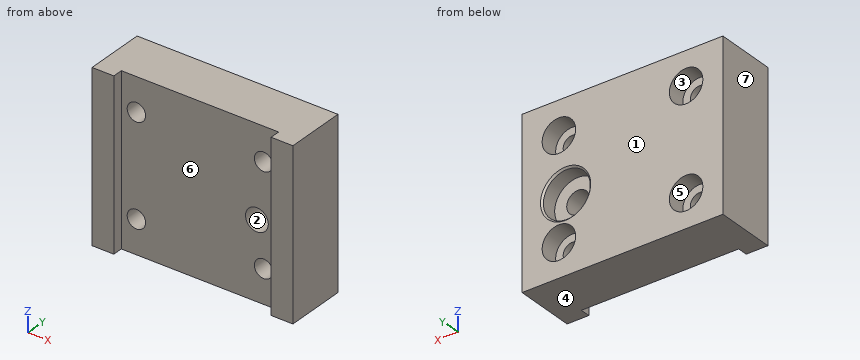
from build123d import *

# Parameters (mm, degrees)
SKETCH1_W                                           = 60
SKETCH1_H                                           = 50
BOSS_EXTRUDE1_DEPTH                                 = 9
SKETCH2_W                                           = 47
SKETCH2_H                                           = 6
CUT_EXTRUDE1_DEPTH                                  = 60
CBORE_FOR_M5_HEX_SOCKET_HEAD_CAP_SCREW1_D           = 5.5
CBORE_FOR_M5_HEX_SOCKET_HEAD_CAP_SCREW1_CBORE_D     = 10
CBORE_FOR_M5_HEX_SOCKET_HEAD_CAP_SCREW1_CBORE_DEPTH = 5.4
M8_TAPPED_HOLE1_D                                   = 6.8
SKETCH9_R                                           = 7
CUT_EXTRUDE2_DEPTH                                  = 5
CHAMFER1_SIZE                                       = 0.5


with BuildPart() as part:
    # Sketch1 → Boss-Extrude1 (new, symmetric)
    with BuildSketch(Plane(origin=(0, 0, 0), x_dir=(1, 0, 0), z_dir=(0, 1, 0))):
        Rectangle(SKETCH1_W, SKETCH1_H)
    extrude(amount=BOSS_EXTRUDE1_DEPTH, both=True)

    # Sketch2 → Cut-Extrude1 (cut, through all)
    with BuildSketch(Plane.XY.offset(25)):
        with Locations((0, -9)):
            Rectangle(SKETCH2_W, SKETCH2_H)
    extrude(amount=-CUT_EXTRUDE1_DEPTH, mode=Mode.SUBTRACT)

    # CBORE for M5 Hex Socket Head Cap Screw1 (through all)
    with Locations(Plane(origin=(0, 9, 0), x_dir=(1, 0, 0), z_dir=(0, 1, 0))):
        with Locations((-19, 15), (19, 15), (19, -15), (-19, -15)):
            CounterBoreHole(CBORE_FOR_M5_HEX_SOCKET_HEAD_CAP_SCREW1_D / 2, CBORE_FOR_M5_HEX_SOCKET_HEAD_CAP_SCREW1_CBORE_D / 2, CBORE_FOR_M5_HEX_SOCKET_HEAD_CAP_SCREW1_CBORE_DEPTH)

    # M8 Tapped Hole1 (through all)
    with Locations(Plane(origin=(0, 9, 0), x_dir=(1, 0, 0), z_dir=(0, 1, 0))):
        with Locations((17, 2)):
            Hole(M8_TAPPED_HOLE1_D / 2)

    # Sketch9 → Cut-Extrude2 (cut)
    with BuildSketch(Plane(origin=(0, 9, 0), x_dir=(1, 0, 0), z_dir=(0, 1, 0))):
        with Locations(Location((17, 2, 0), (0, 0, 270))):
            Circle(SKETCH9_R)
    extrude(amount=-CUT_EXTRUDE2_DEPTH, mode=Mode.SUBTRACT)

    # Chamfer1
    chamfer1_edges = [part.edges().sort_by_distance(p)[0] for p in [
        (17, 9, -9),
    ]]
    chamfer(chamfer1_edges, length=CHAMFER1_SIZE)


solid = part.part
CAD build for the part. Positions are in the model's coordinates, mm. Face numbers are marked on the shaded views. A direction names the side the tool comes from. Round coordinates to 2 decimals unless told otherwise and drop trailing zeros. Loops run counter-clockwise (first coordinate to the right, second up) from the corner with the lowest first, then second, coordinate; pieces in that order, holes last. Notation, with made-up numbers: M 69.25,26 L 122.25,26 A10 ccw 122.25,33 Z; hole C -4.75,34.5 d9. An arc over 180 degrees is marked long. One line per question, with ' | ' between items. Start each with the question number.
Item 1: Cut at B-B, the plane y = -1. Write the cut outline in (x, z).
Item 2: Cut at C-C, the plane z = -2. Write the cut outline in (x, y), plus the area to 3 significant figures.
Item 3: Pin check, flat tips, straight feed: pin 1 Ø6.5 at (x, z) = (19, 15) entering from -Y; pin 2 Ø6 at (x, z) = (17, -2) entering from +Y; pin 3 Ø6.5 at (x, z) = (19, -15) entering from +Y. Stop position of each tip, or through.
Item 4: Two-plate mould, pull along Z, no slides. Class the marked faces 1, 2, 3 and 4: pulls with the +Z half, pulls with the -Z half, needs draft (parallel to the pull), parting line crosses it, or undercut.
Item 5: Wall check: line 1 (Z direction, x = -19, y = -0.25); line 2 (X direction, y = -3.25, z = 15); line 3 (Z direction, x = -19, y = 6.2). Give the ranges that are in metal, low to high.
Item 6: Cut at D-D, the plane x = 17. State how many separate pieces and enclosed holes the cut face has, plus the area to 3 significant figures.
Item 7: Which spindle directions (+Z, -Z, +X, -X, +Y, -Y) get a long thin tool onto all of the face, cutting with end or side? Do the marked faces 5, 6 and 7. Say none if no direction does.
Item 8: Cut at A-A, the plane z = 15. Write the cut outline in (x, y), plus the area to 3 significant figures.
Responses:
1) outline: M -30,-25 L 30,-25 L 30,25 L -30,25 Z; hole C -19,-15 d5.5; hole C -19,15 d5.5; hole C 17,-2 d6.8; hole C 19,-15 d5.5; hole C 19,15 d5.5
2) outline: M -30,-9 L -23.5,-9 L -23.5,-6 L 13.6,-6 L 13.6,4 L 10,4 L 10,8.5 L 9.5,9 L -30,9 Z; M 20.4,-6 L 23.5,-6 L 23.5,-9 L 30,-9 L 30,9 L 24.5,9 L 24,8.5 L 24,4 L 20.4,4 Z | area: 801 mm²
3) pin 1: stops at y = -6 | pin 2: passes through | pin 3: stops at y = 3.6
4) face 1: needs draft | face 2: undercut | face 3: undercut | face 4: pulls with the -Z half
5) line 1: z = -25 to -17.75, -12.25 to 12.25, 17.75 to 25 | line 2: x = -30 to -21.75, -16.25 to 16.25, 21.75 to 30 | line 3: z = -25 to -20, -10 to 10, 20 to 25
6) separate pieces: 4 | enclosed holes: 0 | area: 440 mm²
7) face 5: +Y | face 6: +Z, -Z, -Y | face 7: +Z, -Z, -X, +Y, -Y
8) outline: M -30,-9 L -23.5,-9 L -23.5,-6 L -21.75,-6 L -21.75,3.6 L -24,3.6 L -24,9 L -30,9 Z; M -16.25,-6 L 16.25,-6 L 16.25,3.6 L 14,3.6 L 14,9 L -14,9 L -14,3.6 L -16.25,3.6 Z; M 21.75,-6 L 23.5,-6 L 23.5,-9 L 30,-9 L 30,9 L 24,9 L 24,3.6 L 21.75,3.6 Z | area: 725 mm²
